Solid Edge part; units mm, degrees
sketch "Sketch1" plane through (0, 0, 0) normal (0, -1, 0) x (1, 0, 0)
  line L0 (-2.5, -2.25) -> (2.5, -2.25)
  line L1 (2.5, -2.25) -> (2.5, 2.25)
  line L2 (2.5, 2.25) -> (-2.5, 2.25)
  line L3 (-2.5, 2.25) -> (-2.5, -2.25)
  dimension "D1" = 2.5
  dimension "D2" = 2.5
extrude "Protrusion1" add sketch "Sketch1" along normal mid plane 30
fillet "Round_1" radius 1 1 edges at (2.5, 0, 2.25)
hole "Hole_1" at (-2.5, 7, 0) direction (1, 0, 0) diameter 2 end up to next
mirror "Mirror1" about plane through (0, 0, 0) normal (0, -1, 0) of "Hole_1"
fillet "Round_2" radius 1 5 edges at (-0.5, 15, 2.25) (2.2071, 15, 1.9571) (2.5, 15, -0.5) (-2.5, 15, 0) (0, 15, -2.25)
mirror "Mirror2" about plane through (0, 0, 0) normal (0, -1, 0) of "Round_2"
Geometry check sheet. Reference: the model listing, model coordinates, mm. Round coordinates to 2 decimals unless told otherwise and drop trailing zeros. Write each loop counter-clockwise with the first axis right and the second up, starting at its lowest first coordinate (ties: lowest second). Pieces come first, ordered by that corner, then holes. Notation, with made-up numbers: (43, 60) - (55, 60) arc R19 ccw to (55, 74) - close; hole circle Ø10 at (7.5, 56). An arc over 180 degrees is marked (long way). Write each question's results on one line, items separated by ' | '.
(1) Sectioned sample at D-D, the plane x = 1.85. Enter the section's corners in (y, z), plus the area to 3 significant figures.
Computed:
outline: (-14.94, -1.6) arc R1 ccw to (-14, -2.25) - (14, -2.25) arc R1 ccw to (14.94, -1.6) - (14.94, 1.25) arc R0.94 ccw to (14, 2.19) - (-14, 2.19) arc R0.94 ccw to (-14.94, 1.25) - close; hole circle Ø2 at (-7, 0); hole circle Ø2 at (7, 0) | area: 126 mm^2
(2) Thickness scan on probe 1 along Y at (x, z) = (-0.35, 0); probe 2 along Y at (x, z) = (-2.05, -0.7); probe 3 along Z at (x, y) = (0.65, 7). Record the ranges inside material, lowest first. Write a range as from..to.
Computed:
probe 1: y = -15..-8, -6..6, 8..15 | probe 2: y = -14.84..-7.71, -6.29..6.29, 7.71..14.84 | probe 3: z = -2.25..-1, 1..2.25
(3) Draft check along Z on faces 1 (the face through (-2.5, 0, 0)), 2 (the face through (0, 8, 0)), 3 (the face through (-0.528, -14.715, 1.949)), 4 (the face through (0.035, 14.699, -1.965)). Enter one of: pulls with the +Z half, pulls with the -Z half, needs draft (parallel to the pull), parting line crosses it, or undercut.
Computed:
face 1: needs draft | face 2: undercut | face 3: pulls with the +Z half | face 4: pulls with the -Z half
(4) Sectioned sample at C-C, the plane z = -0.75. Enter the section's corners in (x, y), plus the area to 3 significant figures.
Computed:
outline: (-2.5, -14) arc R1 ccw to (-1.5, -15) - (1.5, -15) arc R1 ccw to (2.5, -14) - (2.5, -7.66) - (-2.5, -7.66) - close; (-2.5, -6.34) - (2.5, -6.34) - (2.5, 6.34) - (-2.5, 6.34) - close; (-2.5, 7.66) - (2.5, 7.66) - (2.5, 14) arc R1 ccw to (1.5, 15) - (-1.5, 15) arc R1 ccw to (-2.5, 14) - close | area: 136 mm^2
(5) Depth check by flat-ended pin: pin 1 Ø1.6 at (y, z) = (7, 0) entering from -X. Enter the tip coordinate at first touch or a pass-through.
Computed:
pin 1: passes through
(6) Sectioned sample at B-B, the plane y = 7. Enter the section's corners in (x, z), plus the area to 3 significant figures.
Computed:
outline: (-2.5, -2.25) - (2.5, -2.25) - (2.5, -1) - (-2.5, -1) - close; (-2.5, 1) - (2.5, 1) - (2.5, 1.25) arc R1 ccw to (1.5, 2.25) - (-2.5, 2.25) - close | area: 12.3 mm^2
(7) Sectioned sample at A-A, the plane x = -0.45. Enter the section's corners in (y, z), plus the area to 3 significant figures.
Computed:
outline: (-15, -1.25) arc R1 ccw to (-14, -2.25) - (14, -2.25) arc R1 ccw to (15, -1.25) - (15, 1.25) arc R1 ccw to (14, 2.25) - (-14, 2.25) arc R1 ccw to (-15, 1.25) - close; hole circle Ø2 at (-7, 0); hole circle Ø2 at (7, 0) | area: 128 mm^2
